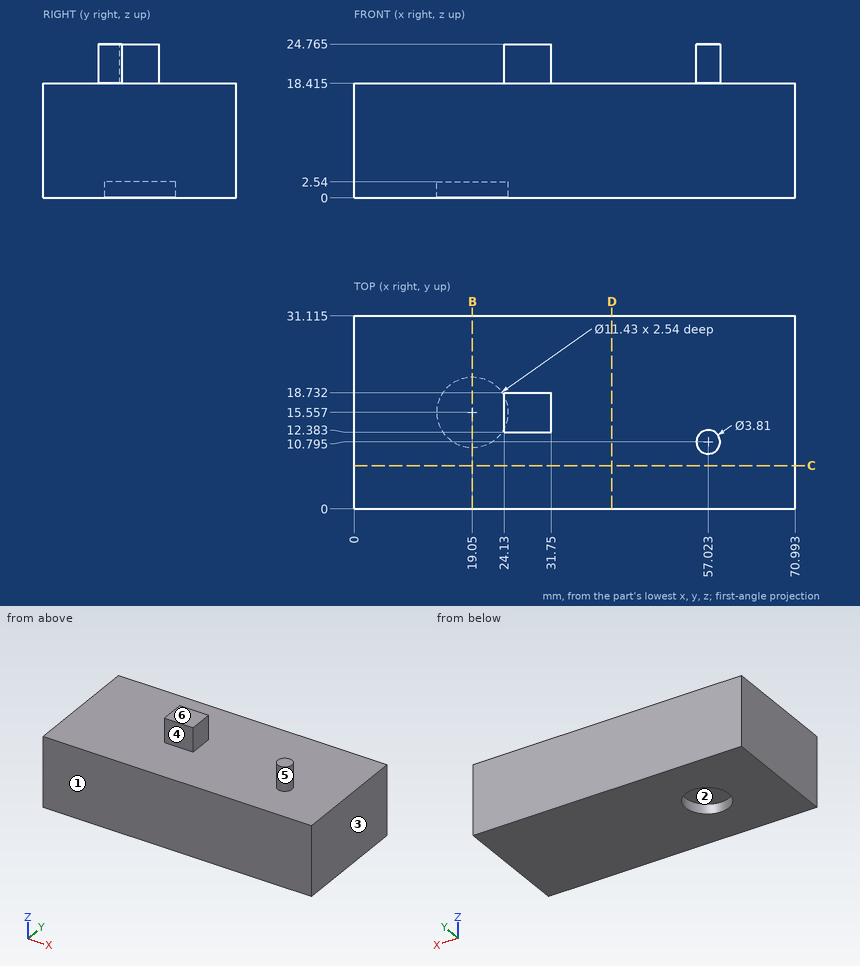
Print and shaded views of the part. All mm, measured from the part's lowest x, y and z. A direction names the side the tool comes from. Coordinates: 2 decimals unless noted, no trailing zeros. Write each loop counter-clockwise with the first axis right and the second up, starting at its lowest first coordinate (ties: lowest second). Pieces come first, ordered by that corner, then holes.
(1) Two-plate mould, pull along X, no slides. Class the marked faces 1, 2 and 3: +X half, -X half, draft (parallel to the pull), parting line (faces both ways), or undercut.
(2) Cut at C-C, the plane y = 7. List the corners of the cut face in (x, z) (1 decimal).
(3) Drill centre lines: probe 1 along Z at (x, y) = (53, 17.5) (1 decimal); probe 2 along Y at (x, z) = (19.05, 1.3) (1 decimal); probe 3 along Z at (x, y) = (21.5, 10.5) (1 decimal). Where is each one in solid material? Low to high.
(4) Cut at D-D, the plane x = 41.5. List the corners of the cut face in (y, z) (1 decimal).
(5) Cut at B-B, the plane x = 19.05. List the corners of the cut face in (y, z) (1 decimal).
(6) 3-axis set-ups, long thin cutter, end or side, ignore diameter. For the marked faces 4, 5 and 6: which of +Z, -Z, +X, -X, +Y, -Y reach the whole face in a straight line?
(7) Flat gauge pins, fed straight in: pin 1 (4 mm diameter, centred on x = 20.5, y = 5.5, fed in from +Z) (1 decimal); pin 2 (7 mm diameter, centred on x = 29, z = 22.5, fed in from -Y); pin 3 (1.5 mm diameter, centred on x = 11, z = 19.5, fed in from +Y); pin 4 (3 mm diameter, centred on y = 14.5, z = 23, fed in from -X). Where does each tip first touch, or does it go through?
Geometry says:
1. face 1: draft
1. face 2: undercut
1. face 3: +X half
2. outline: (0, 0) - (71, 0) - (71, 18.4) - (0, 18.4) - close
3. probe 1: z = 0 to 18.4
3. probe 2: y = 0 to 9.8, 21.3 to 31.1
3. probe 3: z = 2.5 to 18.4
4. outline: (0, 0) - (31.1, 0) - (31.1, 18.4) - (0, 18.4) - close
5. outline: (0, 0) - (9.8, 0) - (9.8, 2.5) - (21.3, 2.5) - (21.3, 0) - (31.1, 0) - (31.1, 18.4) - (0, 18.4) - close
6. face 4: +Z, -X, -Y
6. face 5: +Z
6. face 6: +Z, +X, -X, +Y, -Y
7. pin 1: stops at z = 18.4
7. pin 2: stops at y = 12.38
7. pin 3: passes through
7. pin 4: stops at x = 24.13
